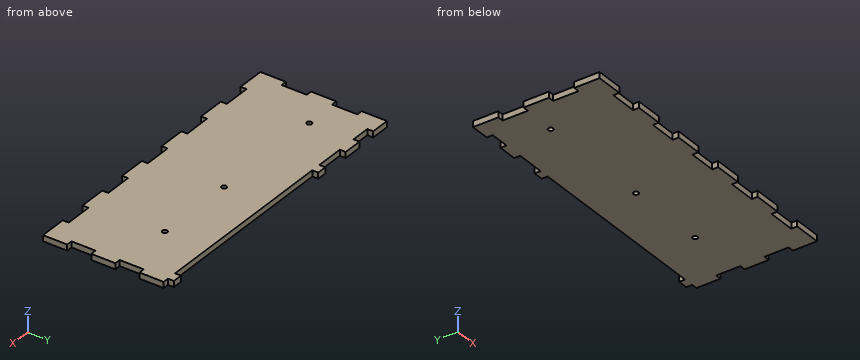
```python
from build123d import *

# Parameters (mm, degrees)
CROQUIS1_R              = 1.25
SALIENTE_EXTRUIR1_DEPTH = 3


with BuildPart() as part:
    # Croquis1 → Saliente-Extruir1 (new body)
    with BuildSketch(Plane.XY):
        Polygon((96.61, -16.741574692), (0, -16.741574692), (0, -13.741574692), (-5, -13.741574692), (-5, -16.741574692), (-9.678, -16.741574692), (-19.356, -16.741574692), (-19.356, -13.741574692), (-29.034, -13.741574692), (-29.034, -16.741574692), (-38.712, -16.741574692), (-38.712, -13.741574692), (-48.39, -13.741574692), (-48.39, -26.541574692), (-45.39, -26.541574692), (-45.39, -39.341574692), (-48.39, -39.341574692), (-48.39, -52.141574692), (-45.39, -52.141574692), (-45.39, -64.941574692), (-48.39, -64.941574692), (-48.39, -77.741574692), (-34.480909091, -77.741574692), (-34.480909091, -74.741574692), (-20.571818182, -74.741574692), (-20.571818182, -77.741574692), (-6.662727273, -77.741574692), (-6.662727273, -74.741574692), (7.246363636, -74.741574692), (7.246363636, -77.741574692), (21.155454545, -77.741574692), (21.155454545, -74.741574692), (35.064545455, -74.741574692), (35.064545455, -77.741574692), (48.973636364, -77.741574692), (48.973636364, -74.741574692), (62.882727273, -74.741574692), (62.882727273, -77.741574692), (76.791818182, -77.741574692), (76.791818182, -74.741574692), (90.700909091, -74.741574692), (90.700909091, -77.741574692), (104.61, -77.741574692), (104.61, -65.541574692), (101.61, -65.541574692), (101.61, -53.341574692), (104.61, -53.341574692), (104.61, -41.141574692), (101.61, -41.141574692), (101.61, -28.941574692), (104.61, -28.941574692), (104.61, -16.741574692), (101.61, -16.741574692), (101.61, -13.741574692), (96.61, -13.741574692), align=None)
        with Locations((-28.49, -38.741574692)):
            Circle(CROQUIS1_R, mode=Mode.SUBTRACT)
        with Locations((31.5, -38.741574692)):
            Circle(CROQUIS1_R, mode=Mode.SUBTRACT)
        with Locations((73.11, -38.741574692)):
            Circle(CROQUIS1_R, mode=Mode.SUBTRACT)
    extrude(amount=SALIENTE_EXTRUIR1_DEPTH)


solid = part.part
```
The model under review builds one solid part; all positions refer to its coordinate system, in mm. Round coordinates to 2 decimals unless told otherwise and drop trailing zeros. Loops run counter-clockwise (first coordinate to the right, second up) from the corner with the lowest first, then second, coordinate; pieces in that order, holes last.
1) Consider section A-A on x = 4. State the section outline as (y, z) points, then the cut area to 3 significant figures.
Values follow:
outline: (-74.74, 0) - (-16.74, 0) - (-16.74, 3) - (-74.74, 3) - close
area: 174 mm2
2) Consider section B-B on y = -35. State the section outline as (x, z) points, then the cut area to 3 significant figures.
Values follow:
outline: (-45.39, 0) - (101.61, 0) - (101.61, 3) - (-45.39, 3) - close
area: 441 mm2
3) Clearance check with flat-ended pins moving along their axes: P1, Ø1.5, axis at x = 26.5, z = 1, coming from the -Y side; P2, Ø1.5, axis at x = -33.5, z = 2, coming from the +Y side. State where each tip first meets the part, or that it passes through.
Values follow:
P1: stops at y = -74.74
P2: stops at y = -16.74
4) Wall thickness on line 1 along Y through (x, z) = (-28.49, 1.8); line 2 along X through (y, z) = (-16.5, 0.55); line 3 along Y through (x, z) = (73.11, 1): over which ranges is each line inside the solid? List them lowest first.
Values follow:
line 1: y = -74.74 to -39.99, -37.49 to -13.74
line 2: x = -48.39 to -38.71, -29.03 to -19.36, -5 to 0, 96.61 to 101.61
line 3: y = -77.74 to -39.99, -37.49 to -16.74
5) Consider section C-C on z = 1.4. Give the number of separate pieces and of enclosed holes in the cut face, then the cut area to 3 significant figures.
Values follow:
separate pieces: 1
enclosed holes: 3
area: 9,050 mm2
